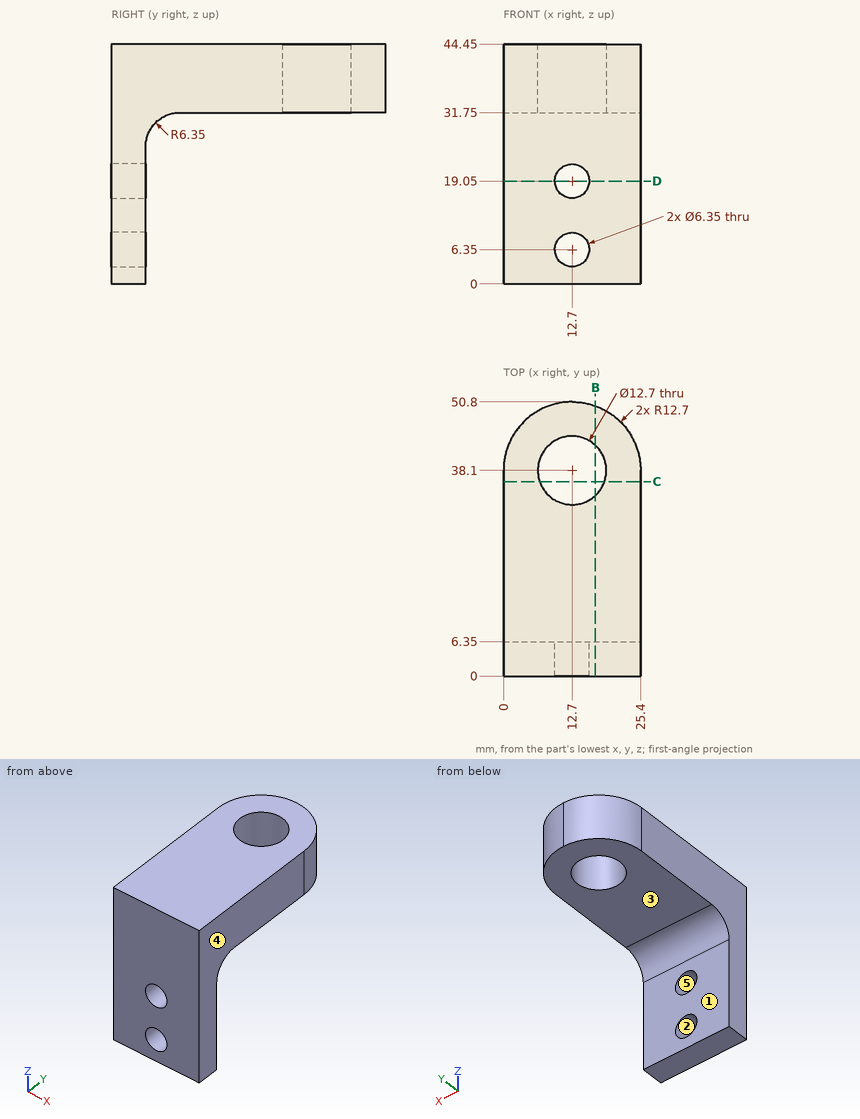
Verification items for this drawing (mm, ordinates from the low corner). A direction names the side the tool comes from. Give positions to 0.01 mm unless a question says otherwise; leave off trailing zeros. Order: outer loops, then holes, each group sorted by start corner. A loop starts at its lowest first (then second) coordinate and runs counter-clockwise, first axis right, second up. Notation, with made-up numbers: M 29,23.5 L 48,23.5 A20 ccw 48,41.5 Z; hole C 24,-20 d11. An arc over 180 degrees is marked long. Use a Markdown table: item, result.
Item 1: Tool access check on the marked faces 1 and 2. Record the directions out of +Z, -Z, +X, -X, +Y, -Y that give a thin tool (end or side, any length) a straight path to the whole face; none if there is none.
Answers follow:
| item | result |
|---|---|
| face 1 | -Z, +X, -X, +Y |
| face 2 | +Y, -Y |
Item 2: Section check D-D (z = 19.05). Record the cut outline in (x, y) (3 decimals), and give its area (3 significant figures).
Answers follow:
| item | result |
|---|---|
| outline | M 0,0 L 9.525,0 L 9.525,6.35 L 0,6.35 Z; M 15.875,0 L 25.4,0 L 25.4,6.35 L 15.875,6.35 Z |
| area | 121 mm2 |
Item 3: Depth check by flat-ended pin: P1, Ø2, axis at x = 14, y = 29, coming from the -Z side. Enter the tip coordinate at first touch or a pass-through.
Answers follow:
| item | result |
|---|---|
| P1 | stops at z = 31.75 |
Item 4: Draft check along Z on the marked faces 3, 4 and 5. Enter one of: +Z half, -Z half, draft (parallel to the pull), parting line (faces both ways), or undercut.
Answers follow:
| item | result |
|---|---|
| face 3 | -Z half |
| face 4 | draft |
| face 5 | undercut |
Item 5: Section check C-C (y = 36). Record the cut outline in (x, z).
Answers follow:
| item | result |
|---|---|
| outline | M 0,31.75 L 6.71,31.75 L 6.71,44.45 L 0,44.45 Z; M 18.69,31.75 L 25.4,31.75 L 25.4,44.45 L 18.69,44.45 Z |
Item 6: Material ranges on line 1 along X through (y, z) = (4, 19); line 2 along Y through (x, z) = (12.7, 37); line 3 along Y through (x, z) = (20.25, 12.5), recorded low to high.
Answers follow:
| item | result |
|---|---|
| line 1 | x = 0 to 9.53, 15.87 to 25.4 |
| line 2 | y = 0 to 31.75, 44.45 to 50.8 |
| line 3 | y = 0 to 6.35 |
Item 7: Section check B-B (x = 17). Record the cut outline in (y, z), and give its area (3 significant figures).
Answers follow:
| item | result |
|---|---|
| outline | M 0,0 L 6.35,0 L 6.35,25.4 A6.35 cw 12.7,31.75 L 33.43,31.75 L 33.43,44.45 L 0,44.45 Z; M 42.77,31.75 L 50.05,31.75 L 50.05,44.45 L 42.77,44.45 Z |
| area | 727 mm2 |
